Here's how the part is built. I have some questions about the finished solid (model axes, mm). A direction names the side the tool comes from. Give positions to 0.01 mm unless a question says otherwise; leave off trailing zeros. Loops run counter-clockwise (first coordinate to the right, second up) from the corner with the lowest first, then second, coordinate; pieces in that order, holes last. Notation, with made-up numbers: (19.25, -11) - (57.25, -11) arc R30 cw to (57.25, 26) - close; hole circle Ø5 at (-10.75, -14). An arc over 180 degrees is marked (long way). Use one line per item in the form item = value.
from build123d import *

# Parameters (mm, degrees)
PAD005_DEPTH           = 3
SKETCH009_W            = 3
SKETCH009_H            = 10
SKETCH009_W_2          = 10
SKETCH009_H_2          = 3
POCKET003_DEPTH        = 3
LINEARPATTERN003_COUNT = 3
LINEARPATTERN003_PITCH = 80
SKETCH011_W            = 10
SKETCH011_H            = 3
SKETCH011_W_2          = 3
SKETCH011_H_2          = 10
POCKET004_DEPTH        = 3


with BuildPart() as part:
    # Sketch008 → Pad005 (new body)
    with BuildSketch(Plane.XZ):
        with BuildLine():
            Line((-3, 260), (-3, 0))
            Line((-3, 0), (7, 0))
            ThreePointArc((14, 7), (9.050253, 4.949747), (7, 0))
            Line((14, 7), (80, 7))
            ThreePointArc((87, 0), (84.949747, 4.949747), (80, 7))
            Line((87, 0), (97, 0))
            Line((97, 0), (97, 260))
            ThreePointArc((97, 260), (85.284271, 288.284271), (57, 300))
            Line((57, 300), (37, 300))
            ThreePointArc((37, 300), (8.715729, 288.284271), (-3, 260))
        make_face()
        with BuildLine():
            ThreePointArc((37, 290), (27, 280), (37, 270))
            Line((37, 270), (57, 270))
            ThreePointArc((57, 270), (67, 280), (57, 290))
            Line((37, 290), (57, 290))
        make_face(mode=Mode.SUBTRACT)
    extrude(amount=PAD005_DEPTH)

    # Sketch009 → Pocket003 (cut)
    with BuildSketch(Plane.XZ.offset(3)):
        with Locations((1.5, 18)):
            Rectangle(SKETCH009_W, SKETCH009_H)
        with Locations((8, 11.5)):
            Rectangle(SKETCH009_W_2, SKETCH009_H_2)
        with Locations((32, 11.5)):
            Rectangle(SKETCH009_W_2, SKETCH009_H_2)
        with Locations((92.5, 23)):
            Rectangle(SKETCH009_W, SKETCH009_H)
    pocket003 = extrude(amount=-POCKET003_DEPTH, mode=Mode.SUBTRACT)

    # LinearPattern003: Pocket003 ×3
    with Locations(*[(0, 0, i * LINEARPATTERN003_PITCH) for i in range(1, LINEARPATTERN003_COUNT)]):
        add(pocket003, mode=Mode.SUBTRACT)

    # Sketch011 → Pocket004 (cut)
    with BuildSketch(Plane.XZ.offset(3)):
        with Locations((8, 248.5)):
            Rectangle(SKETCH011_W, SKETCH011_H)
        with Locations((47, 248.5)):
            Rectangle(SKETCH011_W, SKETCH011_H)
        with Locations((86, 248.5)):
            Rectangle(SKETCH011_W, SKETCH011_H)
        with Locations((1.5, 255)):
            Rectangle(SKETCH011_W_2, SKETCH011_H_2)
        with Locations((92.5, 255)):
            Rectangle(SKETCH011_W_2, SKETCH011_H_2)
    extrude(amount=-POCKET004_DEPTH, mode=Mode.SUBTRACT)


with BuildPart() as part_1:
    # Body005 placement: moved
    add(part.part.moved(Location((0, 0, 3))))


solid = part_1.part
(1) Thinking about a two-plate mould opening in Z: for faces 4 (the flat face through (46, 0, 155)), 5 (the cylindrical face through (27, -1, 283)), 6 (the cylindrical face through (85, -1.5, 7.9)), which applies, pulls with the +Z half, pulls with the -Z half, needs draft (parallel to the pull), parting line crosses it, or undercut?
Geometry says:
face_4 = needs draft
face_5 = undercut
face_6 = pulls with the -Z half
(2) If we section it at A-A (z = 256): List the corners of the cut face in (x, y) for me.
Geometry says:
outline = (-3, -3) - (0, -3) - (0, 0) - (-3, 0) - close; (3, -3) - (91, -3) - (91, 0) - (3, 0) - close; (94, -3) - (97, -3) - (97, 0) - (94, 0) - close
(3) For P1, Ø1.5, axis at x = 33, y = -1, coming from the +Z side; P2, Ø1.5, axis at x = 31.5, y = -1.5, coming from the -Z side; P3, Ø0.9, axis at x = 29.5, y = -1.5, coming from the +Z side, each with a flat end and sliding along its axis, tell me the tip position at first contact or that it passes through.
Geometry says:
P1 = 302.87
P2 = 10
P3 = 302.37
(4) For faces 1 (the flat face through (46, -3, 155)), 2 (the cylindrical face through (9.1, -1.5, 8)), 3 (the cylindrical face through (67, -1, 283)), which set-ups out of +Z, -Z, +X, -X, +Y, -Y let a thin tool reach every point of the face, with its end or its side?
Geometry says:
face_1 = +Z, -Z, +X, -X, -Y
face_2 = -Z, +Y, -Y
face_3 = +Y, -Y
(5) If I drill on probe 1 along Z at (x, y) = (49.5, -2.85); probe 2 along Z at (x, y) = (11.5, -2.2); probe 3 along Z at (x, y) = (40, -0.2), over which ranges is the centre line in solid material (lowest first)?
Geometry says:
probe_1 = 10 to 250, 253 to 273, 293 to 303
probe_2 = 9.54 to 13, 16 to 93, 96 to 173, 176 to 250, 253 to 293.82
probe_3 = 10 to 273, 293 to 303
(6) If we section it at C-C (x = 72.5): List the corners of the cut face in (y, z) for me, plus the area to 3 significant figures.
Geometry says:
outline = (-3, 10) - (0, 10) - (0, 299.87) - (-3, 299.87) - close
area = 870 mm²
